CAD build for the part. Positions are in the model's coordinates, mm. A direction names the side the tool comes from. Round coordinates to 2 decimals unless told otherwise and drop trailing zeros. Write each loop counter-clockwise with the first axis right and the second up, starting at its lowest first coordinate (ties: lowest second). Pieces come first, ordered by that corner, then holes. Notation, with made-up numbers: (11.25, -21) - (19.25, -21) arc R11 ccw to (19.25, -4) - close; hole circle Ø10 at (6.25, 49). An arc over 180 degrees is marked (long way). Use one line per item in the form item = value. Start each with the question number.
Item 1: Pin check, flat tips, straight feed: pin 1 (4 mm diameter, centred on y = 141.5, z = 6.5, fed in from +X); pin 2 (1.5 mm diameter, centred on x = 12.5, z = 3.5, fed in from -Y); pin 3 (3 mm diameter, centred on x = 12, z = 5.5, fed in from -Y). Stop position of each tip, or through.
Item 2: Tool access for faces 1 (the flat face through (-10, 74, 5)), 2 (the flat face through (10, 76, 10)), 3 (the flat face through (30, 74, 5)), 4 (the flat face through (0, 21, 5)): list every direction of +Z, -Z, +X, -X, +Y, -Y with a clear straight run to the whole face (end or side of a thin tool).
Item 3: Drill centre lines: L1, parallel to Y at x = 10, z = 4.5; L2, parallel to X at y = 33.5, z = 2; L3, parallel to X at y = 150, z = 4. Where is each one in solid material? Low to high.
Item 4: Band-saw the part on D-D, the plane x = 18. Give the number of separate pieces and of enclosed holes in the cut face, and give its area (3 significant figures).
Item 5: Band-saw the part on B-B, the plane z = 3.75. List the corners of the cut face in (x, y), and give its area (3 significant figures).
Item 6: Band-saw the part on A-A, the plane x = 10. List the corners of the cut face in (y, z).
Item 7: Band-saw the part on C-C, the plane y = 66. List the corners of the cut face in (x, z).
Item 8: Pull direction Y, two halves, no side cores. Call faces 5 (the flat face through (10, 76, 0)), 6 (the flat face through (10, 40.5, 5)): +Y half, -Y half, draft (parallel to the pull), parting line (faces both ways), or undercut.
Autodesk Inventor part; units mm, degrees
ref_plane "YZ Plane" through (0, 0, 0) normal (1, 0, 0) x (0, 1, 0)
ref_plane "XZ Plane" through (0, 0, 0) normal (0, 1, 0) x (-1, 0, 0)
ref_plane "XY Plane" through (0, 0, 0) normal (0, 0, 1) x (1, 0, 0)
sketch "Sketch1" plane through (0, 0, 0) normal (0, 0, 1) x (1, 0, 0)
  line L0 (0, 0) -> (20, 0)
  line L1 (20, 0) -> (20, 41)
  line L2 (20, 41) -> (0, 41)
  line L3 (0, 41) -> (0, 0)
  circle A0 centre (10, 0) radius 30
  circle A1 centre (10, 0) radius 10
  line L4 (10, 0) -> (30, 0)
  line L5 (30, 0) -> (30, 150)
  line L6 (30, 150) -> (10, 150)
  line L7 (10, 150) -> (10, 0)
  line L8 (10, 0) -> (-10, 0)
  line L9 (-10, 0) -> (-10, 150)
  line L10 (-10, 150) -> (10, 150)
  line L11 (10, 150) -> (10, 0)
  circle A2 centre (10, 150) radius 30
  circle A3 centre (10, 150) radius 10
  point P0 (30, 22.3607)
  point P1 (30, 127.6393)
  point P2 (-10, 127.6393)
  point P3 (-10, 22.3607)
  dimension "d0" = 20
  dimension "d1" = 41
  dimension "d2" = 60
  dimension "d3" = 20
  dimension "d4" = 150
  dimension "d5" = 20
  dimension "d6" = 150
  dimension "d7" = 60
  dimension "d8" = 20
extrude "Extrusion1" add sketch "Sketch1" along normal blind 10 contours L8 L9 A0 L3 | L3 A0 L7 A1 | A1 L4 L5 A0 L9 L8 | A0 L9 A2 L7 L2 L3 | L3 L2 L7 A0 | A1 L7 A0 L1 | L1 A0 L5 L4 | L7 L2 L1 A0 | L1 L2 L7 A2 L5 A0 | A2 L5 L6 A3 L10 L9 | L9 L10 A3 L7 A2 | L7 A3 L6 L5 A2
fillet "Fillet1" radius 2 8 edges at (10, 180, 10) (-10, 75, 10) (10, -30, 10) (10, -30, 0) (-10, 75, 0) (10, 180, 0) (30, 75, 0) (30, 75, 10)
sketch "Sketch2" plane through (0, 0, 10) normal (0, 0, 1) x (1, 0, 0)
  line L0 (0, 0) -> (20, 0)
  line L1 (20, 0) -> (20, 40.5)
  line L2 (20, 40.5) -> (0, 40.5)
  line L3 (0, 40.5) -> (0, 0)
  dimension "d12" = 20
  dimension "d13" = 40.5
extrude "Extrusion2" cut sketch "Sketch2" against normal blind 10.6375
properties part number "First arm"
Determined:
q1.pin_1 = 39.29
q1.pin_2 = -29.95
q1.pin_3 = -30
q2.face_1 = +Z, -Z, -X
q2.face_2 = +Z, +X, -X, +Y, -Y
q2.face_3 = +Z, -Z, +X
q2.face_4 = +Z, -Z
q3.L1 = -30 to -10, 40.5 to 140, 160 to 180
q3.L2 = -10 to 0, 20 to 30
q3.L3 = -20 to 0, 20 to 40
q4.separate_pieces = 3
q4.enclosed_holes = 0
q4.area = 1,490 mm²
q5.outline = (-10, 22.36) arc R30 ccw (long way) to (30, 22.36) - (30, 127.64) arc R30 ccw (long way) to (-10, 127.64) - close; hole (0, 0) arc R10 ccw to (20, 0) - (20, 40.5) - (0, 40.5) - close; hole circle Ø20 at (10, 150)
q5.area = 8,170 mm²
q6.outline = (-30, 2) arc R2 ccw to (-28, 0) - (-10, 0) - (-10, 10) - (-28, 10) arc R2 ccw to (-30, 8) - close; (40.5, 0) - (140, 0) - (140, 10) - (40.5, 10) - close; (160, 0) - (178, 0) arc R2 ccw to (180, 2) - (180, 8) arc R2 ccw to (178, 10) - (160, 10) - close
q7.outline = (-10, 2) arc R2 ccw to (-8, 0) - (28, 0) arc R2 ccw to (30, 2) - (30, 8) arc R2 ccw to (28, 10) - (-8, 10) arc R2 ccw to (-10, 8) - close
q8.face_5 = draft
q8.face_6 = undercut
